Autodesk Inventor part; units mm, degrees
ref_plane "YZ Plane" through (0, 0, 0) normal (1, 0, 0) x (0, 1, 0)
ref_plane "XZ Plane" through (0, 0, 0) normal (0, 1, 0) x (-1, 0, 0)
ref_plane "XY Plane" through (0, 0, 0) normal (0, 0, 1) x (1, 0, 0)
sketch "Sketch2" plane through (0, 0, 0) normal (0, 0, 1) x (1, 0, 0)
  line L0 (0, 0) -> (70, 0)
  line L1 (0, 0) -> (0, 25)
  line L2 (0, 25) -> (40, 25)
  line L3 (40, 25) -> (70, 0)
  dimension "d0" = 70
  dimension "d1" = 25
  dimension "d2" = 40
revolve "Revolution1" add sketch "Sketch2" angle 360 about axis through (0, 0, 0) along (0, 1, 0)
sketch "Sketch3" plane through (0, 25, 0) normal (0, 1, 0) x (1, 0, 0)
  circle A0 centre (0, 0) radius 25
  dimension "d4" = 50
extrude "Extrusion1" add sketch "Sketch3" along normal blind 8
sketch "Sketch4" plane through (0, 33, 0) normal (0, 1, 0) x (1, 0, 0)
  line L0 (-41.5, 38.25) -> (41.5, 38.25)
  line L1 (41.5, 38.25) -> (41.5, -38.25)
  line L2 (41.5, -38.25) -> (-41.5, -38.25)
  line L3 (-41.5, -38.25) -> (-41.5, 38.25)
  point P0 (0, 0)
  point P1 (0, -38.25)
  point P2 (-41.5, 0)
  dimension "d7" = 83
  dimension "d8" = 76.5
extrude "Extrusion2" add sketch "Sketch4" along normal blind 3
properties part number "Pomodoro Robot Base"
Verification items for the finished model (mm, model axes). Give positions to 0.01 mm unless a question says otherwise; leave off trailing zeros. Loops run counter-clockwise (first coordinate to the right, second up) from the corner with the lowest first, then second, coordinate; pieces in that order, holes last.
1. Material ranges on probe 1 along Y at (x, z) = (-7, -31.5); probe 2 along X at (y, z) = (34, 1.5); probe 3 along Y at (x, z) = (-35, 27.5), recorded low to high.
Derived:
probe 1: y = 0 to 25, 33 to 36
probe 2: x = -41.5 to 41.5
probe 3: y = 0 to 21.24, 33 to 36
2. Cross-section at D-D on y = 4. Record the cut outline in (x, z).
Derived:
outline: circle Ø130.4 at (0, 0)
3. Release check for a two-part mould opening along Y. For faces 1 (the flat face through (-1, 36, -1)), 2 (the flat face through (17.22, 25, -18.34)), 3 (the flat face through (-1, 0, -1)) record: +Y half, -Y half, draft (parallel to the pull), parting line (faces both ways), or undercut.
Derived:
face 1: +Y half
face 2: undercut
face 3: -Y half
4. Cross-section at B-B on x = 0. Record the cut outline in (y, z).
Derived:
outline: (0, -70) - (25, -40) - (25, -25) - (33, -25) - (33, -38.25) - (36, -38.25) - (36, 38.25) - (33, 38.25) - (33, 25) - (25, 25) - (25, 40) - (0, 70) - close
5. Cross-section at C-C on y = 22.5. Record the cut outline in (x, z).
Derived:
outline: circle Ø86 at (0, 0)
6. Cross-section at A-A on z = 0. Record the cut outline in (x, y).
Derived:
outline: (-70, 0) - (70, 0) - (40, 25) - (25, 25) - (25, 33) - (41.5, 33) - (41.5, 36) - (-41.5, 36) - (-41.5, 33) - (-25, 33) - (-25, 25) - (-40, 25) - close
7. Go/stop test with flat-tipped pins: P1, Ø1.5, axis at x = 43.5, y = 13.5, coming from the -Z side; P2, Ø10, axis at x = -10, y = 32.5, coming from the -Z side; P3, Ø3, axis at x = -18, z = 45, coming from the -Y side; P4, Ø3, axis at x = 11, y = 6.5, coming from the -Z side. Record where each tip stops, or that it passes through.
Derived:
P1: stops at z = -33.46
P2: stops at z = -38.25
P3: stops at y = 0
P4: stops at z = -63.07
